Can you work these out from the model? Positions are in its coordinate system, mm. Face numbers are marked on the shaded views. A direction names the side the tool comes from. Give positions to 0.01 mm unless a question says otherwise; leave off trailing zeros. Order: outer loops, then holes, each group sorted by start corner. A loop starts at its lowest first (then second) coordinate and runs counter-clockwise, first axis right, second up. Notation, with made-up numbers: (86, 13.25) - (144, 13.25) arc R14 ccw to (144, 17.25) - close; hole circle Ø8 at (81.5, 25.25). An arc over 180 degrees is marked (long way). Answer as CSV lines item,"result".
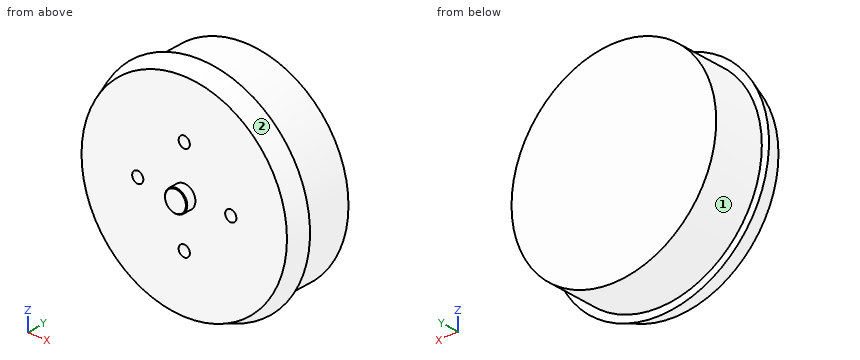
```python
from build123d import *

# Parameters (mm, degrees)
SKETCH1_R           = 29.5
BOSS_EXTRUDE1_DEPTH = 5
SKETCH2_R           = 27.5
BOSS_EXTRUDE2_DEPTH = 14
CHAMFER1_SIZE       = 5.220207097
CHAMFER1_SIZE_2     = 1.9
SKETCH3_R           = 1.5
CUT_EXTRUDE1_DEPTH  = 3.5
SKETCH4_R           = 3
BOSS_EXTRUDE3_DEPTH = 2.7
CHAMFER2_SIZE       = 0.2


with BuildPart() as part:
    # Sketch1 → Boss-Extrude1 (new body)
    with BuildSketch(Plane(origin=(0, 0, 0), x_dir=(1, 0, 0), z_dir=(0, 1, 0))):
        with Locations(Location((0, 0, 0), (0, 0, 270))):
            Circle(SKETCH1_R)
    extrude(amount=BOSS_EXTRUDE1_DEPTH)

    # Sketch2 → Boss-Extrude2 (add)
    with BuildSketch(Plane(origin=(0, 5, 0), x_dir=(1, 0, 0), z_dir=(0, 1, 0))):
        with Locations(Location((0, 0, 0), (0, 0, 270))):
            Circle(SKETCH2_R)
    extrude(amount=BOSS_EXTRUDE2_DEPTH)

    # Chamfer1
    # the kernel refuses this chamfer: 5.220207097, 1.9 mm, written as the material it takes off along each edge
    with BuildSketch(Plane(origin=(0, 0, 0), x_dir=(0, 0, 1), z_dir=(-1, 0, 0))) as chamfer1_piece_1:
        Polygon((29.5, CHAMFER1_SIZE), (29.5 - CHAMFER1_SIZE_2, 0), (29.5, 0), align=None)
    revolve(axis=Axis((0, 0, 0), (0, 1, 0)), mode=Mode.SUBTRACT)

    # Sketch3 → Cut-Extrude1 (cut)
    with BuildSketch(Plane.XZ):
        with Locations(Location((0, 12.5, 0), (0, 0, 270))):
            Circle(SKETCH3_R)
        with Locations(Location((12.5, 0, 0), (0, 0, 270))):
            Circle(SKETCH3_R)
        with Locations(Location((0, -12.5, 0), (0, 0, 270))):
            Circle(SKETCH3_R)
        with Locations(Location((-12.5, 0, 0), (0, 0, 270))):
            Circle(SKETCH3_R)
    extrude(amount=-CUT_EXTRUDE1_DEPTH, mode=Mode.SUBTRACT)

    # Sketch4 → Boss-Extrude3 (add)
    with BuildSketch(Plane.XZ):
        with Locations(Location((0, 0, 0), (0, 0, 90))):
            Circle(SKETCH4_R)
    extrude(amount=BOSS_EXTRUDE3_DEPTH)

    # Chamfer2
    chamfer2_edges = [part.edges().sort_by_distance(p)[0] for p in [
        (0, -2.7, -3),
    ]]
    chamfer(chamfer2_edges, length=CHAMFER2_SIZE)


solid = part.part
```
1) I want a section at A-A on z = 0. Write out the boundary of the cut face in (x, y).
Answer block:
outline,"(-29.42, 5) - (-27.6, 0) - (-14, 0) - (-14, 3.5) - (-11, 3.5) - (-11, 0) - (-3, 0) - (-3, -2.5) - (-2.8, -2.7) - (2.8, -2.7) - (3, -2.5) - (3, 0) - (11, 0) - (11, 3.5) - (14, 3.5) - (14, 0) - (27.6, 0) - (29.42, 5) - (27.5, 5) - (27.5, 19) - (-27.5, 19) - (-27.5, 5) - close"
2) I want a section at B-B on x = 0. Write out the boundary of the cut face in (y, z).
Answer block:
outline,"(-2.7, -2.8) - (-2.5, -3) - (0, -3) - (0, -11) - (3.5, -11) - (3.5, -14) - (0, -14) - (0, -27.6) - (5, -29.42) - (5, -27.5) - (19, -27.5) - (19, 27.5) - (5, 27.5) - (5, 29.42) - (0, 27.6) - (0, 14) - (3.5, 14) - (3.5, 11) - (0, 11) - (0, 3) - (-2.5, 3) - (-2.7, 2.8) - close"
3) I need wall thicknesses on line 1 along X through (y, z) = (1.5, 0); line 2 along X through (y, z) = (2.15, 0); line 3 along Y through (x, z) = (-8, 14.5). Which ranges of each line are inside material? Lowest first, please. Write a range as [from, to].
Answer block:
line 1,"[-28.15, -14], [-11, 11], [14, 28.15]"
line 2,"[-28.38, -14], [-11, 11], [14, 28.38]"
line 3,"[0, 19]"
4) I'm going to push flat-ended pins straight in: P1, Ø2.5, axis at x = 0.5, z = 13, coming from the -Y side; P2, Ø1.5, axis at x = 13, z = -0.5, coming from the -Y side; P3, Ø3, axis at y = 11.5, z = -0.5, coming from the +X side. Where does each tip first touch, or does it pass through?
Answer block:
P1,"y = 0"
P2,"y = 3.5"
P3,"x = 27.5"
5) I want a section at C-C on y = 7.5. Write out the boundary of the cut face in (x, z), plus the area to 3 significant figures.
Answer block:
outline,"circle Ø55 at (0, 0)"
area,"2,380 mm2"
6) Which directions (+Z, -Z, +X, -X, +Y, -Y) give clear straight access to the entire face, cutting with the end or side of a thin tool? Please do the marked faces 1 and 2.
Answer block:
face 1,"+Y"
face 2,"-Y"
